```python
from build123d import *

# Parameters (mm, degrees)
F0_R     = 3.175
F0_R_2   = 3.96875
F1_DEPTH = 3.175
F2_R     = 7.9375


with BuildPart() as f1:
    # F0 (on Top) → F1 (new body)
    with BuildSketch(Plane.XY):
        with BuildLine():
            ThreePointArc((-44.7334821429, -7.9324362036), (-38.9384772185, -5.7120069047), (-36.5125, 0))
            ThreePointArc((-36.5125, 0), (-38.9384772185, 5.7120069047), (-44.7334821429, 7.9324362036))
            ThreePointArc((-44.7334821429, 7.9324362036), (-52.3875, 0), (-44.7334821429, -7.9324362036))
        make_face()
        with Locations((-44.45, 0)):
            Circle(F0_R, mode=Mode.SUBTRACT)
        with BuildLine():
            ThreePointArc((-44.7334821429, 7.9324362036), (-38.9384772185, 5.7120069047), (-36.5125, 0))
            ThreePointArc((-36.5125, 0), (-38.9384772185, -5.7120069047), (-44.7334821429, -7.9324362036))
            Line((-44.7334821429, -7.9324362036), (-0.3401785714, -9.5189234444))
            ThreePointArc((-0.3401785714, -9.5189234444), (-6.5286582423, -6.9355783144), (-9.481007206, -0.9144))
            Line((-9.481007206, -0.9144), (-10.4524001899, 9.157542126))
            Line((-10.4524001899, 9.157542126), (-44.7334821429, 7.9324362036))
        make_face()
        with BuildLine():
            Line((-0.3401786498, 9.5189234416), (-10.4524001899, 9.157542126))
            Line((-10.4524001899, 9.157542126), (-9.481007206, -0.9144))
            ThreePointArc((-9.481007206, -0.9144), (-7.1643200942, 6.2767939736), (-0.3401786498, 9.5189234416))
        make_face()
        with BuildLine():
            Line((-15.5488518178, 62.000384), (-10.4524001899, 9.157542126))
            Line((-10.4524001899, 9.157542126), (-0.3401786498, 9.5189234416))
            ThreePointArc((-0.3401786498, 9.5189234416), (6.6138273095, 6.8544083129), (9.525, 0))
            ThreePointArc((9.525, 0), (9.5139954445, -0.4577288296), (9.481007206, -0.9144))
            Line((9.481007206, -0.9144), (15.5488518178, 62.000384))
            ThreePointArc((15.5488518178, 62.000384), (0, 47.879), (-15.5488518178, 62.000384))
        make_face()
        with Locations((0, 20.6502)):
            Circle(F0_R, mode=Mode.SUBTRACT)
        with BuildLine():
            ThreePointArc((-9.481007206, -0.9144), (-6.5286582423, -6.9355783144), (-0.3401785714, -9.5189234444))
            ThreePointArc((-0.3401785714, -9.5189234444), (6.2767940031, -7.1643200684), (9.481007206, -0.9144))
            ThreePointArc((9.481007206, -0.9144), (9.5139954445, -0.4577288296), (9.525, 0))
            ThreePointArc((9.525, 0), (6.6138273095, 6.8544083129), (-0.3401786498, 9.5189234416))
            ThreePointArc((-0.3401786498, 9.5189234416), (-7.1643200942, 6.2767939736), (-9.481007206, -0.9144))
        make_face()
        Circle(F0_R_2, mode=Mode.SUBTRACT)
        with BuildLine():
            ThreePointArc((15.621, 63.5), (-0.7506752806, 79.102952529), (-15.5488518178, 62.000384))
            ThreePointArc((-15.5488518178, 62.000384), (0, 47.879), (15.5488518178, 62.000384))
            ThreePointArc((15.5488518178, 62.000384), (15.602952529, 62.7493247194), (15.621, 63.5))
        make_face()
        with Locations((0, 63.5)):
            Circle(F0_R_2, mode=Mode.SUBTRACT)
    extrude(amount=F1_DEPTH)

    # F2
    f2_edges = [f1.edges().sort_by_distance(p)[0] for p in [
        (-10.4524, 9.157542, 1.5875),
    ]]
    fillet(f2_edges, radius=F2_R)


solid = f1.part
```
Can you work these out from the model? Positions are in its coordinate system, mm. A direction names the side the tool comes from. Coordinates: 2 decimals unless noted, no trailing zeros. Loops run counter-clockwise (first coordinate to the right, second up) from the corner with the lowest first, then second, coordinate; pieces in that order, holes last. Notation, with made-up numbers: (47, 62) -> (103, 62) arc R27 ccw to (103, 100) -> close; hole circle Ø5 at (7, 11). An arc over 180 degrees is marked (long way). Put each result on its own line as item: value. Start each with the question number.
Q1. I want a section at C-C (x = -39). Write out the boundary of the cut face in (y, z) (3 decimals).
Q2. I want a section at D-D (y = 41). Write out the boundary of the cut face in (x, z) (3 decimals).
Q3. Thinking about a two-plate mould opening in Y: for faces 1 (the face through (-0.517, 67.435, 1.565)), 2 (the face through (-0.4, 23.8, 1.6)), 3 (the face through (-11, 26, 3.175)), 4 (the face through (12.472, 30.103, 1.565)), which applies, pulls with the +Y half, pulls with the -Y half, needs draft (parallel to the pull), parting line crosses it, or undercut?
Q4. I want a section at B-B (z = 2.35). Count the separate pieces of the cut face and the enclosed holes in it, plus the area to 3 significant figures.
Q5. For faces 5 (the face through (-0.86, -3.874, 1.565)), 6 (the face through (-13.435, 40.087, 1.565)), which set-ups out of +Z, -Z, +X, -X, +Y, -Y let a thin tool reach every point of the face, with its end or its side?
Q6. I'm going to push flat-ended pins straight in: P1, Ø1, axis at x = -38, z = 2, coming from the +Y side; P2, Ø1, axis at x = -2.5, z = 0.5, coming from the -Y side; P3, Ø1.5, axis at y = 1, z = 2.5, coming from the +X side. Where does each tip first touch, or does it pass through?
Q7. I want a section at A-A (y = 0). Write out the boundary of the cut face in (x, z) (1 decimal), plus the area to 3 significant figures.
Q8. If I drill on line 1 (Y direction, x = 0, z = 2.3) (3 decimals); line 2 (Y direction, x = -44.45, z = 0.75) (3 decimals); line 3 (X direction, y = -0.5, z = 2.05), over which ranges is the centre line in solid material (lowest first)? Write a range as [from, to].
Taken from the geometry:
1. outline: (-8.137, 0) -> (8.137, 0) -> (8.137, 3.175) -> (-8.137, 3.175) -> close
2. outline: (-13.523, 0) -> (13.523, 0) -> (13.523, 3.175) -> (-13.523, 3.175) -> close
3. face 1: undercut
3. face 2: undercut
3. face 3: needs draft
3. face 4: pulls with the -Y half
4. separate pieces: 1
4. enclosed holes: 4
4. area: 2,690 mm2
5. face 5: +Z, -Z
5. face 6: +Z, -Z, -X
6. P1: stops at y = 8.19
6. P2: stops at y = -9.46
6. P3: stops at x = 9.74
7. outline: (-52.4, 0) -> (-47.6, 0) -> (-47.6, 3.2) -> (-52.4, 3.2) -> close; (-41.3, 0) -> (-4, 0) -> (-4, 3.2) -> (-41.3, 3.2) -> close; (4, 0) -> (9.6, 0) -> (9.6, 3.2) -> (4, 3.2) -> close
7. area: 151 mm2
8. line 1: y = [-9.525, -3.969], [3.969, 17.475], [23.825, 59.531], [67.469, 79.121]
8. line 2: y = [-7.943, -3.175], [3.175, 7.943]
8. line 3: x = [-52.37, -47.59], [-41.31, -3.94], [3.94, 9.52]
